Autodesk Inventor part; units mm, degrees
ref_plane "YZ Plane" through (0, 0, 0) normal (1, 0, 0) x (0, 1, 0)
ref_plane "XZ Plane" through (0, 0, 0) normal (0, 1, 0) x (-1, 0, 0)
ref_plane "XY Plane" through (0, 0, 0) normal (0, 0, 1) x (1, 0, 0)
sketch "Sketch1" plane through (0, 0, 0) normal (1, 0, 0) x (0, 1, 0)
  line L0 (0, 0) -> (0, 38) construction
  line L1 (7, 0) -> (47, 0)
  line L2 (0, 0) -> (7, 0)
  line L3 (7, 0) -> (47, 0)
  line L4 (47, 0) -> (47, 28)
  line L5 (7, 28) -> (7, 0)
  line L6 (47, 28) -> (54, 28) construction
  line L7 (54, 0) -> (54, 47.2) construction
  line L8 (54, 47.2) -> (0, 47.2) construction
  line L9 (0, 28) -> (0, 31.6)
  line L10 (54, 31.6) -> (54, 28)
  line L11 (7, 31.6) -> (7, 37.25)
  line L12 (7, 37.25) -> (47, 37.25)
  line L13 (47, 37.25) -> (47, 31.6)
  line L14 (0, 31.6) -> (7, 31.6)
  line L15 (47, 31.6) -> (54, 31.6)
  line L16 (54, 28) -> (47, 28)
  line L17 (7, 28) -> (0, 28)
  dimension "d0" = 38
  dimension "d1" = 54
  dimension "d3" = 40
  dimension "d4" = 28
  dimension "d5" = 47.2
  dimension "d6" = 3.6
  dimension "d7" = 5.65
  dimension "d49" = 28
  dimension "d50" = 5.65
  dimension "d51" = 3.6
extrude "Extrusion1" add sketch "Sketch1" along normal blind 20
sketch "Sketch2" plane through (0, 7, 37.25) normal (0, 0, 1) x (1, 0, 0)
  line L0 (0, 40) -> (0, 0)
  line L1 (0, 0) -> (20, 0)
  line L2 (20, 40) -> (20, 0)
  line L3 (0, 40) -> (20, 40)
  line L4 (10, 39.7) -> (10, 30)
  line L5 (0, 0) -> (0, 40)
  circle A0 centre (10, 30) radius 1.3
  circle A1 centre (10, 30) radius 3
  arc A2 (19.7, 27.569) -> (0.3, 27.569) centre (10, 30) ccw
  line L6 (19.7, 27.569) -> (19.7, 6.969)
  line L7 (0.3, 6.969) -> (0.3, 27.569)
  arc A3 (5.5, 6.969) -> (14.5, 6.969) centre (10, 11.0315) ccw
  line L8 (19.7, 6.969) -> (14.5, 6.969)
  line L9 (5.5, 6.969) -> (0.3, 6.969)
  line L10 (10, 6.969) -> (10, 4.969) construction
  point P0 (0, -7)
  dimension "d11" = 9.7
  dimension "d12" = 2.6
  dimension "d13" = 6
  dimension "d14" = 20.6
  dimension "d19" = 9
  dimension "d20" = 2
extrude "Extrusion2" add sketch "Sketch2" along normal blind 2.5 contours A2 L6 L8 A3 L9 L7 | A0 | A1
sketch "Sketch3" plane through (0, 7, 39.75) normal (0, 0, 1) x (1, 0, 0)
  line L0 (14.5, 6.969) -> (19.7, 6.969)
  line L1 (0.3, 6.969) -> (0.3, 27.569)
  line L2 (19.7, 6.969) -> (0.3, 6.969)
  line L3 (0.3, 6.969) -> (0.3, 19.669)
  line L4 (19.7, 19.669) -> (19.7, 6.969)
  arc A0 (11.875, 19.669) -> (8.125, 19.669) centre (10, 20.6147) ccw
  line L5 (8.125, 19.669) -> (0.3, 19.669)
  line L6 (11.875, 19.669) -> (19.7, 19.669)
  point P0 (0, -7)
  dimension "d21" = 12.7
  dimension "d25" = 2.1
  dimension "d26" = 3.75
extrude "Extrusion3" add sketch "Sketch3" along normal blind 0.5
sketch "Sketch4" plane through (0, 7, 39.75) normal (0, 0, 1) x (1, 0, 0)
  line L0 (11.875, 19.669) -> (19.7, 19.669)
  line L1 (19.7, 19.669) -> (19.7, 27.569)
  arc A0 (19.7, 27.569) -> (0.3, 27.569) centre (10, 30) ccw
  line L2 (0.3, 27.569) -> (0.3, 19.669)
  line L3 (0.3, 19.669) -> (8.125, 19.669)
  arc A1 (11.875, 19.669) -> (8.125, 19.669) centre (10, 20.6147) ccw
  circle A2 centre (10, 30) radius 6.5
  point P0 (0, -7)
  dimension "d29" = 13
extrude "Extrusion4" add sketch "Sketch4" along normal blind 1 contours A2
sketch "Sketch5" plane through (10, 37, 40.75) normal (0, 0, 1) x (1, 0, 0)
  circle A0 centre (0, 0) radius 5.25
  point P0 (-10, -37)
  dimension "d32" = 10.5
extrude "Extrusion5" add sketch "Sketch5" along normal blind 0.4
sketch "Sketch6" plane through (10, 37, 41.15) normal (0, 0, 1) x (1, 0, 0)
  circle A0 centre (0, 0) radius 2.75
  circle A1 centre (0, 0) radius 1.3
  point P0 (-10, -37)
  dimension "d35" = 5.5
  dimension "d36" = 2.6
extrude "Extrusion6" add sketch "Sketch6" along normal blind 4.3
sketch "Sketch7" plane through (0, 0, 31.6) normal (0, 0, 1) x (1, 0, 0)
  line L0 (0, 7) -> (0, 0)
  line L1 (0, 0) -> (20, 0)
  line L2 (20, 7) -> (20, 0)
  line L3 (0, 7) -> (20, 7)
  line L4 (0, 54) -> (0, 47)
  line L5 (0, 47) -> (20, 47)
  line L6 (20, 54) -> (20, 47)
  line L7 (0, 54) -> (20, 54)
  line L8 (0, 0) -> (3, 0)
  arc A0 (5.5, 0) -> (3, 0) centre (4.25, 1.7493) ccw
  line L9 (10, 0) -> (10, 5.7084)
  arc A1 (17, 0) -> (14.5, 0) centre (15.75, 1.7493) ccw
  line L10 (17, 0) -> (14.5, 0)
  line L11 (0, 7) -> (0, 47)
  line L12 (0, 27) -> (24.9803, 27)
  line L13 (0, 54) -> (20, 54)
  line L14 (0, 54) -> (20, 54)
  line L15 (3, 54) -> (5.5, 54)
  arc A2 (3, 54) -> (5.5, 54) centre (4.25, 52.2507) ccw
  arc A3 (14.5, 54) -> (17, 54) centre (15.75, 52.2507) ccw
  line L16 (17, 54) -> (14.5, 54)
  line L17 (5.5, 54) -> (3, 54)
  line L18 (0, 54) -> (20, 54)
  line L19 (5.5, 0) -> (3, 0)
  point P0 (14.5, 54)
  point P1 (5.5, 54)
  point P2 (3, 54)
  point P3 (17, 0)
  point P4 (14.5, 0)
  point P5 (5.5, 0)
  point P6 (3, 0)
  dimension "d39" = 3
  dimension "d40" = 2.5
  dimension "d42" = 2.15
  dimension "d44" = 2.5
  dimension "d45" = 2.15
extrude "Extrusion7" cut sketch "Sketch7" against normal up to surface (3.6 mm away) contours A0 L1 | L1 A1 | L7 A2 | A3 L7
fillet "Fillet1" radius 1 4 edges at (0, 0, 29.8) (20, 0, 29.8) (0, 54, 29.8) (20, 54, 29.8)
properties part number "Motor Mg995"
Model file for the job. Use its own axes, mm. A direction names the side the tool comes from. Give positions to 0.01 mm unless a question says otherwise; leave off trailing zeros. Write each loop counter-clockwise with the first axis right and the second up, starting at its lowest first coordinate (ties: lowest second). Pieces come first, ordered by that corner, then holes. Notation, with made-up numbers: M 31,-23.75 L 56,-23.75 A16 ccw 56,1.25 Z; hole C 19,18.5 d3. An arc over 180 degrees is marked long. One line per item, written item: value. Start each with the question number.
Q1. Saw through at C-C, the plane z = 6.5. Write the cut outline in (x, y), plus the area to 3 significant figures.
Q2. 3-axis set-ups, long thin cutter, end or side, ignore diameter. For faces 1 (the flat face through (10, 4, 28)), 2 (the flat face through (10, 13, 39.75)), 3 (the flat face through (10, 50, 28)), 4 (the cylindrical face through (9.642, 34.273, 43.27)), 5 (the cylindrical face through (10.07, 11.97, 38.48)): which of +Z, -Z, +X, -X, +Y, -Y reach the whole face in a straight line?
Q3. Drop flat-ended pins along their axis: pin 1 Ø4 at (x, z) = (6.5, 9.5) entering from +Y; pin 2 Ø6 at (x, z) = (9, 15.5) entering from -Y; pin 3 Ø1.5 at (x, z) = (10.5, 38.5) entering from -Y. Give the stop position or say it passes through.
Q4. Saw through at D-D, the plane y = 29. Write the cut outline in (x, z).
Q5. Two-plate mould, pull along Y, no slides. Class faces 6 (the cylindrical face through (10.699, 35.904, 43.27)), 7 (the flat face through (2, 0, 30)), 8 (the flat face through (10, 50, 31.6)): +Y half, -Y half, draft (parallel to the pull), parting line (faces both ways), or undercut.
Q6. Probe probe 1 along Y at (x, z) = (6.75, 9); probe 2 along Z at (x, y) = (4.75, 35); probe 3 along Z at (x, y) = (18, 19). List the from-to ranges inside material, lowest first. Write a range as [from, to].
Q7. Saw through at A-A, the plane y = 22.5. Write the cut outline in (x, z).
Output values:
1. outline: M 0,7 L 20,7 L 20,47 L 0,47 Z
1. area: 800 mm²
2. face 1: -Z, +X, -X, -Y
2. face 2: +Z, +X, -X, -Y
2. face 3: -Z, +X, -X, +Y
2. face 4: +Z
2. face 5: +Z, -Y
3. pin 1: stops at y = 47
3. pin 2: stops at y = 7
3. pin 3: stops at y = 11.97
4. outline: M 0,0 L 20,0 L 20,37.25 L 19.7,37.25 L 19.7,39.75 L 11.58,39.75 L 11.58,40.25 L 8.42,40.25 L 8.42,39.75 L 0.3,39.75 L 0.3,37.25 L 0,37.25 Z
5. face 6: undercut
5. face 7: -Y half
5. face 8: draft
6. probe 1: y = [7, 47]
6. probe 2: z = [0, 40.75]
6. probe 3: z = [0, 40.25]
7. outline: M 0,0 L 20,0 L 20,37.25 L 19.7,37.25 L 19.7,40.25 L 0.3,40.25 L 0.3,37.25 L 0,37.25 Z
